from build123d import *

# Parameters (mm, degrees)
BASE_4_R              = 1.5
BASE_4_R_2            = 0.75
BOSS_EXTRUDE5_DEPTH   = 3
BOSS_EXTRUDE5_2_DEPTH = 3
BASE_W                = 13.5
BASE_H                = 1
BOSS_EXTRUDE7_DEPTH   = 6.5
BASE_7_R              = 1.5
BASE_7_R_2            = 3
BOSS_EXTRUDE8_DEPTH   = 1
BOSS_EXTRUDE9_DEPTH   = 3
SLIT_W                = 10
SLIT_H                = 2
CUT_EXTRUDE2_DEPTH    = 6.5
BASE_13_W             = 4
BASE_13_H             = 1
BOSS_EXTRUDE12_DEPTH  = 9
BOSS_EXTRUDE13_DEPTH  = 4
CUT_EXTRUDE3_DEPTH    = 4
BASE_14_W             = 4
BASE_14_H             = 1
BOSS_EXTRUDE14_DEPTH  = 9


with BuildPart() as part:
    # Base_4 → Boss-Extrude5 (new body)
    with BuildSketch(Plane(origin=(0, 0, 0), x_dir=(1, 0, 0), z_dir=(0, 1, 0))):
        with Locations(Location((-12, -12, 0), (0, 0, 270))):
            Circle(BASE_4_R)
        with Locations(Location((-12, -12, 0), (0, 0, 270))):
            Circle(BASE_4_R_2, mode=Mode.SUBTRACT)
    extrude(amount=BOSS_EXTRUDE5_DEPTH)



with BuildPart() as body_2:
    # Base_4 → Boss-Extrude5 2 (new body)
    with BuildSketch(Plane(origin=(0, 0, 0), x_dir=(1, 0, 0), z_dir=(0, 1, 0))):
        with Locations(Location((12, -12, 0), (0, 0, 270))):
            Circle(BASE_4_R)
        with Locations(Location((12, -12, 0), (0, 0, 270))):
            Circle(BASE_4_R_2, mode=Mode.SUBTRACT)
    extrude(amount=BOSS_EXTRUDE5_2_DEPTH)


with BuildPart() as body_3:
    # Base → Boss-Extrude7 (new body)
    with BuildSketch(Plane(origin=(0, 0, 0), x_dir=(1, 0, 0), z_dir=(0, 1, 0))):
        with Locations((0, 16)):
            Rectangle(BASE_W, BASE_H)
    extrude(amount=BOSS_EXTRUDE7_DEPTH)


with BuildPart() as part_1:
    add(part.part)

    add(body_2.part)  # Boss-Extrude8 merges body 2

    add(body_3.part)  # Boss-Extrude8 merges body 3
    # Base_7 → Boss-Extrude8 (add)
    with BuildSketch(Plane(origin=(0, 0, 0), x_dir=(1, 0, 0), z_dir=(0, 1, 0))):
        with BuildLine():
            ThreePointArc((14, 15), (13.560660172, 16.060660172), (12.5, 16.5))
            Line((12.5, 16.5), (6.75, 16.5))
            Line((6.75, 16.5), (6.75, 15.5))
            Line((6.75, 15.5), (-6.75, 15.5))
            Line((-6.75, 15.5), (-6.75, 16.5))
            Line((-6.75, 16.5), (-12.5, 16.5))
            ThreePointArc((-12.5, 16.5), (-13.560660172, 16.060660172), (-14, 15))
            Line((-14, 15), (-14, -15))
            ThreePointArc((-14, -15), (-13.560660172, -16.060660172), (-12.5, -16.5))
            Line((-12.5, -16.5), (-2, -16.5))
            Line((-2, -16.5), (-2, -15.5))
            Line((-2, -15.5), (2, -15.5))
            Line((2, -15.5), (2, -16.5))
            Line((2, -16.5), (12.5, -16.5))
            ThreePointArc((12.5, -16.5), (13.560660172, -16.060660172), (14, -15))
            Line((14, -15), (14, 15))
        make_face()
        with Locations(Location((-12, -12, 0), (0, 0, 270))):
            Circle(BASE_7_R, mode=Mode.SUBTRACT)
        with Locations(Location((0, -5, 0), (0, 0, 270))):
            Circle(BASE_7_R_2, mode=Mode.SUBTRACT)
        with Locations(Location((12, -12, 0), (0, 0, 270))):
            Circle(BASE_7_R, mode=Mode.SUBTRACT)
        with Locations(Location((0, 5, 0), (0, 0, 270))):
            Circle(BASE_7_R_2, mode=Mode.SUBTRACT)
    extrude(amount=BOSS_EXTRUDE8_DEPTH)

    # Base_8 → Boss-Extrude9 (add)
    with BuildSketch(Plane(origin=(0, 0, 0), x_dir=(1, 0, 0), z_dir=(0, 1, 0))):
        with BuildLine():
            Line((-5, -9.5), (5, -9.5))
            ThreePointArc((5, -9.5), (5.5, -10), (5, -10.5))
            Line((5, -10.5), (-5, -10.5))
            ThreePointArc((-5, -10.5), (-5.5, -10), (-5, -9.5))
        make_face()
        with BuildLine():
            Line((-5, 10.5), (5, 10.5))
            ThreePointArc((5, 10.5), (5.5, 10), (5, 9.5))
            Line((5, 9.5), (-5, 9.5))
            ThreePointArc((-5, 9.5), (-5.5, 10), (-5, 10.5))
        make_face()
    extrude(amount=BOSS_EXTRUDE9_DEPTH)

    # slit → Cut-Extrude2 (cut)
    with BuildSketch(Plane.XY.offset(-15.5)):
        with Locations((0, 4)):
            Rectangle(SLIT_W, SLIT_H)
    extrude(amount=-CUT_EXTRUDE2_DEPTH, mode=Mode.SUBTRACT)

    # Base_13 → Boss-Extrude12 (add)
    with BuildSketch(Plane(origin=(0, 0, 0), x_dir=(1, 0, 0), z_dir=(0, 1, 0))):
        with Locations((0, -16)):
            Rectangle(BASE_13_W, BASE_13_H)
    extrude(amount=BOSS_EXTRUDE12_DEPTH)

    # Sketch3 → Boss-Extrude13 (add)
    with BuildSketch(Plane(origin=(2, 0, 0), x_dir=(0, 0, -1), z_dir=(1, 0, 0))):
        Polygon((-15.5, 7), (-14, 7), (-15.5, 9), align=None)
    extrude(amount=-BOSS_EXTRUDE13_DEPTH)

    # Sketch4 → Cut-Extrude3 (cut)
    with BuildSketch(Plane(origin=(2, 0, 0), x_dir=(0, 0, -1), z_dir=(1, 0, 0))):
        Polygon((-14, 7), (-16.5, 9), (-13.837162957, 9), align=None)
    extrude(amount=-CUT_EXTRUDE3_DEPTH, mode=Mode.SUBTRACT)

    # Base_14 → Boss-Extrude14 (add)
    with BuildSketch(Plane(origin=(0, 0, 0), x_dir=(1, 0, 0), z_dir=(0, 1, 0))):
        with Locations((0, -17)):
            Rectangle(BASE_14_W, BASE_14_H)
    extrude(amount=BOSS_EXTRUDE14_DEPTH)


solid = part_1.part
Work out the finished part from the listing and answer in its coordinate system (mm). A direction names the side the tool comes from. Coordinates: 2 decimals unless noted, no trailing zeros. Write each loop counter-clockwise with the first axis right and the second up, starting at its lowest first coordinate (ties: lowest second). Pieces come first, ordered by that corner, then holes. Notation, with made-up numbers: M 33,77 L 54,77 A22 cw 54,92 Z; hole C 22.5,32 d10. An arc over 180 degrees is marked long. Answer as CSV lines item,"result". Start each with the question number.
Item 1: Section A-A on y = 1.5 is taken. Write down the section's boundary in (x, z), and give its area (3 significant figures).
Item 2: Section D-D on z = 5 is taken. Write down the section's boundary in (x, y).
Item 3: Section C-C on z = 12 is taken. Write down the section's boundary in (x, y).
Item 4: Consider L1, parallel to X at y = 2.4, z = 12; L2, parallel to X at y = 0.95, z = 12; L3, parallel to Z at x = -0.5, y = 1.75. Determine where each line is inside the solid, lowest interval first.
Item 5: Determine the mould class of faces 1 (the face through (-13.57, 0.49, 16.05)), 2 (the face through (0, 9, 17)), 3 (the face through (0.9, 0.49, -2.14)), 4 (the face through (5.5, 2, -10)) for opening direction X: released by +X, released by -X, zero draft, split by the parting line, or undercut.
Item 6: A tool of negligible diameter and unlimited length cuts with its end or side. For faces 5 (the face through (-5.5, 2, -10)), 6 (the face through (12.07, 1.99, 10.5)), 7 (the face through (0, 2, -9.5)), 8 (the face through (0, 3, -16)), from which of +Z, -Z, +X, -X, +Y, -Y can it reach the whole face along a straight path? Write none if from no direction.
Item 7: Section B-B on x = -12 is taken. Write down the section's boundary in (y, z), and give its area (3 significant figures).
Item 8: Flat-ended cylindrical pins translate along their axes: P1, Ø2, axis at x = 12, z = 12, coming from the +Y side; P2, Ø1.5, axis at x = 10.5, y = 4, coming from the +Z side; P3, Ø1.1, axis at y = 5, z = -16, coming from the -X side; P4, Ø1.8, axis at y = 4.5, z = 16.5, coming from the -X side. Find the tip coordinate at first contact, or state that the pin passes through.
Checks:
1,outline,"C -12,12 d3; M -6.75,-16.5 L 6.75,-16.5 L 6.75,-15.5 L -6.75,-15.5 Z; M -5,-10.5 L 5,-10.5 A0.5 ccw 5,-9.5 L -5,-9.5 A0.5 ccw Z; M -5,9.5 L 5,9.5 A0.5 ccw 5,10.5 L -5,10.5 A0.5 ccw Z; M -2,15.5 L 2,15.5 L 2,17.5 L -2,17.5 Z; C 12,12 d3; hole C -12,12 d1.5; hole C 12,12 d1.5"
1,area,"53.7 mm²"
2,outline,"M -14,0 L -3,0 L -3,1 L -14,1 Z; M 3,0 L 14,0 L 14,1 L 3,1 Z"
3,outline,"M -14,0 L -12.75,0 L -12.75,3 L -13.5,3 L -13.5,1 L -14,1 Z; M -11.25,0 L 11.25,0 L 11.25,3 L 10.5,3 L 10.5,1 L -10.5,1 L -10.5,3 L -11.25,3 Z; M 12.75,0 L 14,0 L 14,1 L 13.5,1 L 13.5,3 L 12.75,3 Z"
4,L1,"x = -13.5 to -12.75, -11.25 to -10.5, 10.5 to 11.25, 12.75 to 13.5"
4,L2,"x = -14 to -12.75, -11.25 to 11.25, 12.75 to 14"
4,L3,"z = -16.5 to -15.5, -10.5 to -9.5, 9.5 to 10.5, 15.5 to 17.5"
5,face 1,"released by -X"
5,face 2,"zero draft"
5,face 3,"undercut"
5,face 4,"released by +X"
6,face 5,"-X, +Y"
6,face 6,"+Y"
6,face 7,"+X, -X, +Y"
6,face 8,"-Z"
7,outline,"M 0,-16.5 L 1,-16.5 L 1,10.5 L 3,10.5 L 3,11.25 L 0,11.25 Z; M 0,12.75 L 3,12.75 L 3,13.5 L 1,13.5 L 1,16.5 L 0,16.5 Z"
7,area,"34.5 mm²"
8,P1,"stops at y = 3"
8,P2,"passes through"
8,P3,"stops at x = -6.75"
8,P4,"stops at x = -2"
